For this review, use the dimensioned drawing (mm, ordinates from the lowest corner) and the shaded views. A direction names the side the tool comes from. Coordinates: 2 decimals unless noted, no trailing zeros. Loops run counter-clockwise (first coordinate to the right, second up) from the corner with the lowest first, then second, coordinate; pieces in that order, holes last. Notation, with made-up numbers: M 7.25,37.25 L 15.25,37.25 A3 cw 15.25,42.25 Z; hole C 9,20.5 d8. An arc over 180 degrees is marked long. Write item = value, one per line. Start each with the question number.
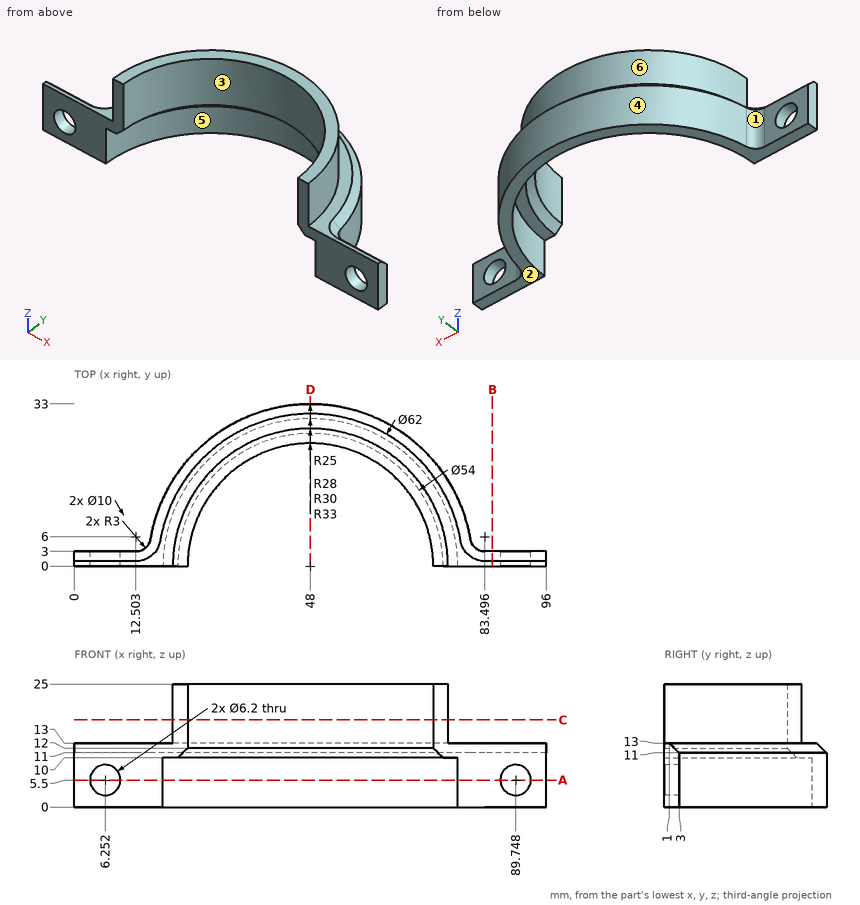
Q1. Mouldability with a two-part tool opening along X and no side actions: class the marked faces 1, 2 and 3 as released by +X, released by -X, zero draft, split by the parting line, or undercut.
Q2. For the marked faces 4, 5 and 6, list the 3-axis set-ups (+Z, -Z, +X, -X, +Y, -Y) from which the entire face can be reached by the end or side of a thin tool; tool diameter is ignored.
Q3. To check wall thickness, follow line 1 (Z direction, x = 74, y = 13.5); line 2 (X direction, y = 25, z = 3) (1 decimal); line 3 (X direction, y = 14, z = 14.25). State the ranges of each line that lie inside material, in increasing order. Write a range as from..to.
Q4. Add section A-A on z = 5.5. State the section outline as (x, y) points.
Q5. Clearance check with flat-ended pins moving along their axes: P1, Ø1.5, axis at y = 21, z = 9, coming from the +X side (1 decimal); P2, Ø1.5, axis at x = 23.5, y = 12, coming from the -Z side; P3, Ø10, axis at x = 89.75, z = 5.5, coming from the -Y side; P4, Ø4, axis at y = 16.5, z = 11, coming from the -X side. State where each tip first meets the part, or that it passes through.
Q6. Add section C-C on z = 17.75. State the section outline as (x, y) points.
Q7. Add section B-B on x = 85. State the section outline as (y, z) points, plus the area to 3 significant figures.
Q8. Add section D-D on x = 48. State the section outline as (y, z) points.
Values follow:
q1.face_1 = released by -X
q1.face_2 = zero draft
q1.face_3 = undercut
q2.face_4 = +Z, -Z, +Y
q2.face_5 = -Z, -Y
q2.face_6 = +Z, +Y
q3.line_1 = 10..13
q3.line_2 = 26.5..31.4, 64.6..69.5
q3.line_3 = 23.75..27.29, 68.71..72.25
q4.outline = M 0,0 L 3.15,0 L 3.15,3 L 0,3 Z; M 9.35,0 L 18,0 A30 cw 78,0 L 86.65,0 L 86.65,3 L 83.5,3 A3 cw 80.54,5.5 A33 ccw 15.46,5.5 A3 cw 12.5,3 L 9.35,3 Z; M 92.85,0 L 96,0 L 96,3 L 92.85,3 Z
q5.P1 = 74.1
q5.P2 = 10
q5.P3 = 0
q5.P4 = 18.36
q6.outline = M 20,0 L 23,0 A25 cw 73,0 L 76,0 A28 ccw Z
q7.outline = M 0,0 L 3,0 L 3,11 L 1,13 L 0,13 Z
q7.area = 37.0 mm2
q8.outline = M 25,12 L 27,10 L 30,10 L 30,0 L 33,0 L 33,11 L 31,13 L 28,13 L 28,25 L 25,25 Z
